```python
from build123d import *

# Parameters (mm, degrees)
SKETCH1_R           = 25
BOSS_EXTRUDE1_DEPTH = 52.5
SKETCH2_R           = 2.5
CUT_EXTRUDE1_DEPTH  = 10
SKETCH3_R           = 20
BOSS_EXTRUDE2_DEPTH = 150
CUT_EXTRUDE2_START  = -5
SKETCH4_R           = 2.5
CUT_EXTRUDE2_DEPTH  = 5


with BuildPart() as part:
    # Sketch1 → Boss-Extrude1 (new, symmetric)
    with BuildSketch(Plane.XY):
        Circle(SKETCH1_R)
    boss_extrude1 = extrude(amount=BOSS_EXTRUDE1_DEPTH, both=True)

    # Sketch2 → Cut-Extrude1 (cut)
    with BuildSketch(Plane(origin=(0, 0, -52.5), x_dir=(-1, 0, 0), z_dir=(0, 0, -1))):
        Circle(SKETCH2_R)
    cut_extrude1 = extrude(amount=-CUT_EXTRUDE1_DEPTH, mode=Mode.SUBTRACT)

    # Sketch3 → Boss-Extrude2 (add)
    with BuildSketch(Plane(origin=(0, 0, 0), x_dir=(1, 0, 0), z_dir=(0, 1, 0))):
        with Locations(Location((0, 0, 0), (0, 0, 90))):
            Circle(SKETCH3_R)
    extrude(amount=BOSS_EXTRUDE2_DEPTH)

    # Mirror1: Boss-Extrude1, Cut-Extrude1 across plane
    add(boss_extrude1.mirror(Plane.ZX.offset(75)))
    add(cut_extrude1.mirror(Plane.ZX.offset(75)), mode=Mode.SUBTRACT)

    # Sketch4 → Cut-Extrude2 (cut)
    with BuildSketch(Plane.XY.offset(52.5).offset(CUT_EXTRUDE2_START)):
        with Locations(Location((0, 150, 0), (0, 0, 180))):
            Circle(SKETCH4_R)
    extrude(amount=CUT_EXTRUDE2_DEPTH, mode=Mode.SUBTRACT)


solid = part.part
```
Model file for the job. Use its own axes, mm. A direction names the side the tool comes from. Coordinates: 2 decimals unless noted, no trailing zeros. Write each loop counter-clockwise with the first axis right and the second up, starting at its lowest first coordinate (ties: lowest second). Pieces come first, ordered by that corner, then holes. Notation, with made-up numbers: (78, 54) - (128, 54) arc R14 cw to (128, 62) - close; hole circle Ø9 at (38.5, 88). An arc over 180 degrees is marked (long way). One line per item, written item: value. Start each with the question number.
1. Mould opens along X. For faces 1 (the cylindrical face through (-5.42, 174.406, 0.735)), 2 (the cylindrical face through (0.33, 147.52, -47.57)), 3 (the flat face through (0, 155, 52.5)) say: released by +X, released by -X, zero draft, split by the parting line, or undercut.
2. Slice it at C-C (y = 61). Write the cut outline in (x, z), plus the area to 3 significant figures.
3. Probe line 1 (Y direction, x = 0, z = 50.95); line 2 (Y direction, x = 0, z = -46); line 3 (X direction, y = 150, z = -47.5). List the from-to ranges inside material, lowest first. Write a range as from..to.
4. Slice it at A-A (x = 0). Write the cut outline in (y, z), plus the area to 3 significant figures.
5. Slice it at B-B (z = 38). Write the cut outline in (x, y).
6. Slice it at D-D (z = 0). Write the cut outline in (x, y), plus the area to 3 significant figures.
7. Tool access for faces 4 (the cylindrical face through (-5.42, -24.406, 0.735)), 5 (the flat face through (0, 150, -42.5)), 6 (the cylindrical face through (0.33, 147.52, 49.96)): list every direction of +Z, -Z, +X, -X, +Y, -Y with a clear straight run to the whole face (end or side of a thin tool).
8. Flat gauge pins, fed straight in: pin 1 (1.5 mm diameter, centred on x = 0, y = 0.5, fed in from -Z); pin 2 (5.5 mm diameter, centred on x = 0, y = 150.5, fed in from -Z); pin 3 (12 mm diameter, centred on x = -10.5, y = 115, fed in from +Z); pin 4 (4 mm diameter, centred on x = 0, y = 150, fed in from +Z). Where does each tip first touch, or does it go through?
Answers below:
1. face 1: split by the parting line
1. face 2: undercut
1. face 3: zero draft
2. outline: circle Ø40 at (0, 0)
2. area: 1,260 mm^2
3. line 1: y = -25..25, 125..147.5, 152.5..175
3. line 2: y = -25..-2.5, 2.5..25, 125..147.5, 152.5..175
3. line 3: x = -25..-2.5, 2.5..25
4. outline: (-25, -52.5) - (-2.5, -52.5) - (-2.5, -42.5) - (2.5, -42.5) - (2.5, -52.5) - (25, -52.5) - (25, -20) - (125, -20) - (125, -52.5) - (147.5, -52.5) - (147.5, -42.5) - (152.5, -42.5) - (152.5, -52.5) - (175, -52.5) - (175, 52.5) - (152.5, 52.5) - (152.5, 47.5) - (147.5, 47.5) - (147.5, 52.5) - (125, 52.5) - (125, 20) - (25, 20) - (25, 52.5) - (-25, 52.5) - close
4. area: 14,400 mm^2
5. outline: circle Ø50 at (0, 0); circle Ø50 at (0, 150)
6. outline: (-20, 15) arc R25 ccw (long way) to (20, 15) - (20, 135) arc R25 ccw (long way) to (-20, 135) - close
6. area: 8,170 mm^2
7. face 4: none
7. face 5: -Z
7. face 6: +Z
8. pin 1: stops at z = -42.5
8. pin 2: stops at z = -52.5
8. pin 3: stops at z = 19.49
8. pin 4: stops at z = 47.5
